from build123d import *

# Parameters (mm, degrees)
SKETCH_1_W              = 140
SKETCH_1_H              = 45
SKETCH_1_R              = 4.1
SKETCH_1_R_2            = 0.5
EXTRUDE_1_DEPTH         = 6
M3_TAPPED_HOLE5_D       = 2.5
M3_TAPPED_HOLE2_D       = 2.5
HOLE_WIZARD_4_2_4_2_1_D = 4.2


with BuildPart() as part:
    # 草图1 → 凸台-拉伸1 (new body)
    with BuildSketch(Plane(origin=(0, 0, 0), x_dir=(1, 0, 0), z_dir=(0, 1, 0))):
        Rectangle(SKETCH_1_W, SKETCH_1_H)
        with Locations((60, 0)):
            Circle(SKETCH_1_R, mode=Mode.SUBTRACT)
        with Locations((-60, 0)):
            Circle(SKETCH_1_R, mode=Mode.SUBTRACT)
        with Locations((-40, 15)):
            Circle(SKETCH_1_R_2, mode=Mode.SUBTRACT)
        with Locations((40, 15)):
            Circle(SKETCH_1_R_2, mode=Mode.SUBTRACT)
        with Locations((40, -15)):
            Circle(SKETCH_1_R_2, mode=Mode.SUBTRACT)
        with Locations((-40, -15)):
            Circle(SKETCH_1_R_2, mode=Mode.SUBTRACT)
    extrude(amount=EXTRUDE_1_DEPTH)

    # M3 Tapped Hole5 (through all)
    with Locations(Plane(origin=(0, 6, 0), x_dir=(1, 0, 0), z_dir=(0, 1, 0))):
        with Locations((-40, 15), (-40, -15), (40, -15), (40, 15)):
            Hole(M3_TAPPED_HOLE5_D / 2)

    # M3 Tapped Hole2 (through all)
    with Locations(Plane(origin=(0, 6, 0), x_dir=(1, 0, 0), z_dir=(0, 1, 0))):
        with Locations((-21.5, 13.5), (21.5, 13.5), (21.5, -18.5), (-21.5, -18.5)):
            Hole(M3_TAPPED_HOLE2_D / 2)

    # Ø4.2 (4.2) 直径孔1 (through all)
    with Locations(Plane(origin=(0, 6, 0), x_dir=(1, 0, 0), z_dir=(0, 1, 0))):
        with Locations((50, 0), (-50, 0)):
            Hole(HOLE_WIZARD_4_2_4_2_1_D / 2)


solid = part.part
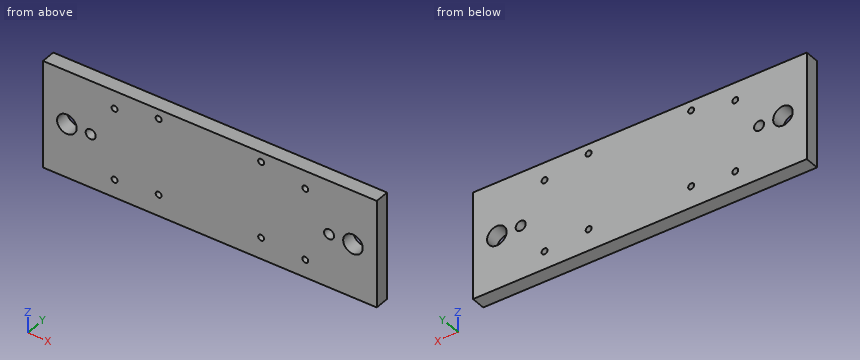
Geometry check sheet. Reference: the model listing, model coordinates, mm. Round coordinates to 2 decimals unless told otherwise and drop trailing zeros. Loops run counter-clockwise (first coordinate to the right, second up) from the corner with the lowest first, then second, coordinate; pieces in that order, holes last.
Item 1: Cross-section at A-A on x = -60. Record the boundary of the cut face in (y, z), then the cut area to 3 significant figures.
Item 2: Thickness scan on line 1 (Z direction, x = -40, y = 1.65); line 2 (X direction, y = 2.5, z = 18.5); line 3 (Z direction, x = 21.5, y = 1.45). Record the ranges inside material, lowest first.
Item 3: Cross-section at B-B on y = 1.45. Count the separate pieces of the cut face and the enclosed holes in it, then the cut area to 3 significant figures.
Item 4: Cross-section at D-D on z = 0. Record the boundary of the cut face in (x, y).
Item 5: Cross-section at C-C on x = -40. Record the boundary of the cut face in (y, z).
Item 6: Gauge pin test, flat ends, axial feed: pin 1 (3 mm diameter, centred on x = 40, z = -15, fed in from -Y); pin 2 (7.5 mm diameter, centred on x = 60, z = 0, fed in from -Y). Record the tip position at first contact, or that the pin passes through.
Answer sheet:
1. outline: (0, -22.5) - (6, -22.5) - (6, -4.1) - (0, -4.1) - close; (0, 4.1) - (6, 4.1) - (6, 22.5) - (0, 22.5) - close
1. area: 221 mm2
2. line 1: z = -22.5 to -16.25, -13.75 to 13.75, 16.25 to 22.5
2. line 2: x = -70 to -22.75, -20.25 to 20.25, 22.75 to 70
2. line 3: z = -22.5 to -14.75, -12.25 to 17.25, 19.75 to 22.5
3. separate pieces: 1
3. enclosed holes: 12
3. area: 6,130 mm2
4. outline: (-70, 0) - (-64.1, 0) - (-64.1, 6) - (-70, 6) - close; (-55.9, 0) - (-52.1, 0) - (-52.1, 6) - (-55.9, 6) - close; (-47.9, 0) - (47.9, 0) - (47.9, 6) - (-47.9, 6) - close; (52.1, 0) - (55.9, 0) - (55.9, 6) - (52.1, 6) - close; (64.1, 0) - (70, 0) - (70, 6) - (64.1, 6) - close
5. outline: (0, -22.5) - (6, -22.5) - (6, -16.25) - (0, -16.25) - close; (0, -13.75) - (6, -13.75) - (6, 13.75) - (0, 13.75) - close; (0, 16.25) - (6, 16.25) - (6, 22.5) - (0, 22.5) - close
6. pin 1: stops at y = 0
6. pin 2: passes through
